The model under review builds one solid part; all positions refer to its coordinate system, in mm. A direction names the side the tool comes from. Give positions to 0.01 mm unless a question says otherwise; leave off trailing zeros. Order: outer loops, then holes, each group sorted by start corner. A loop starts at its lowest first (then second) coordinate and runs counter-clockwise, first axis right, second up. Notation, with made-up numbers: (-10.75, 48) - (6.25, 48) arc R18 cw to (6.25, 80) - close; hole circle Ø11 at (55, 84.5). An arc over 180 degrees is marked (long way). Put each result on its own line as item: value.
```python
from build123d import *

# Parameters (mm, degrees)
F0_R     = 3.175
F0_R_2   = 9.525
F1_DEPTH = 25.4
F2_R     = 5.08
F3_SIZE  = 1.5875
F4_R     = 1.5875
F5_SIZE  = 1.5875


with BuildPart() as f1:
    # F0 (on Top) → F1 (new body)
    with BuildSketch(Plane.XY):
        Polygon((0, 0), (-25.4, 0), (-25.4, -25.4), (50.8, -25.4), (50.8, 38.1), (25.4, 38.1), (25.4, 12.7), (0, 12.7), align=None)
        with Locations((-12.7, -12.7)):
            Circle(F0_R, mode=Mode.SUBTRACT)
        with Locations((25.4, 0)):
            Circle(F0_R_2, mode=Mode.SUBTRACT)
    extrude(amount=F1_DEPTH)

    # F2
    f2_edges = [f1.edges().sort_by_distance(p)[0] for p in [
        (50.8, 38.1, 12.7),
        (25.4, 38.1, 12.7),
        (25.4, 12.7, 12.7),
        (0, 12.7, 12.7),
        (0, 0, 12.7),
        (-25.4, 0, 12.7),
        (-25.4, -25.4, 12.7),
        (50.8, -25.4, 12.7),
    ]]
    fillet(f2_edges, radius=F2_R)

    # F3
    f3_edges = [f1.edges().sort_by_distance(p)[0] for p in [
        (15.875, 0, 25.4),
    ]]
    chamfer(f3_edges, length=F3_SIZE)

    # F4
    f4_edges = [f1.edges().sort_by_distance(p)[0] for p in [
        (-25.4, -12.7, 25.4),
        (12.7, -25.4, 0),
    ]]
    fillet(f4_edges, radius=F4_R)

    # F5
    f5_edges = [f1.edges().sort_by_distance(p)[0] for p in [
        (15.875, 0, 0),
    ]]
    chamfer(f5_edges, length=F5_SIZE)


solid = f1.part
```
(1) Take a section at D-D, the plane y = 20.5. Write out the cut boundary in (x, z) (1 decimal), then the cut area to 3 significant figures.
The answers:
outline: (25.4, 1.6) arc R1.6 ccw to (27, 0) - (49.2, 0) arc R1.6 ccw to (50.8, 1.6) - (50.8, 23.8) arc R1.6 ccw to (49.2, 25.4) - (27, 25.4) arc R1.6 ccw to (25.4, 23.8) - close
area: 643 mm^2
(2) Take a section at B-B, the plane y = -12.7. Write out the cut boundary in (x, z) (1 decimal).
The answers:
outline: (-25.4, 1.6) arc R1.6 ccw to (-23.8, 0) - (-15.9, 0) - (-15.9, 25.4) - (-23.8, 25.4) arc R1.6 ccw to (-25.4, 23.8) - close; (-9.5, 0) - (49.2, 0) arc R1.6 ccw to (50.8, 1.6) - (50.8, 23.8) arc R1.6 ccw to (49.2, 25.4) - (-9.5, 25.4) - close
(3) The part is to be moulded in two halves that separate along X. For faces 5 (the cylindrical face through (-23.872, -1.449, 12.856)), 6 (the cylindrical face through (15.884, 0.419, 12.544)), 7 (the cylindrical face through (50.35, 6.72, 0.48)), say which applies: pulls with the +X half, pulls with the -X half, needs draft (parallel to the pull), parting line crosses it, or undercut.
The answers:
face 5: pulls with the -X half
face 6: undercut
face 7: pulls with the +X half
(4) For faces 1 (the cylindrical face through (-12.81, -0.48, 24.95)), 2 (the flat face through (13, 12.7, 13)), 3 (the cylindrical face through (-12.81, -0.45, 0.48)), 4 (the cylindrical face through (13.16, -24.95, 0.48)), list the 3-axis set-ups (+Z, -Z, +X, -X, +Y, -Y) from which the entire face can be reached by the end or side of a thin tool; tool diameter is ignored.
The answers:
face 1: +Z, -X, +Y
face 2: +Z, -Z, -X, +Y
face 3: -Z, -X, +Y
face 4: -Z, +X, -X, -Y
(5) Take a section at C-C, the plane x = -12.7. Write out the cut boundary in (y, z) (1 decimal).
The answers:
outline: (-25.4, 1.6) arc R1.6 ccw to (-23.8, 0) - (-15.9, 0) - (-15.9, 25.4) - (-23.8, 25.4) arc R1.6 ccw to (-25.4, 23.8) - close; (-9.5, 0) - (-1.6, 0) arc R1.6 ccw to (0, 1.6) - (0, 23.8) arc R1.6 ccw to (-1.6, 25.4) - (-9.5, 25.4) - close
(6) Clearance check with flat-ended pins moving along their axes: pin 1 Ø12 at (x, z) = (-14.5, 12.5) entering from +Y; pin 2 Ø3 at (y, z) = (6.5, 8.5) entering from -X; pin 3 Ø4.5 at (y, z) = (22.5, 7.5) entering from -X; pin 4 Ø15 at (x, y) = (25.4, 0) entering from -Z. State where each tip first meets the part, or that it passes through.
The answers:
pin 1: y = 0
pin 2: x = 0
pin 3: x = 25.4
pin 4: through
(7) Wall thickness on L1, parallel to Y at x = -12.7, z = 8.25 (3 decimals); L2, parallel to Y at x = 10, z = 19.5; L3, parallel to X at y = 4.5, z = 19.5: over which ranges is each line inside the solid? List them lowest first.
The answers:
L1: -25.4 to -15.875, -9.525 to 0
L2: -25.4 to 12.7
L3: -0.03 to 17.01, 33.79 to 50.8
(8) Take a section at A-A, the plane z = 6.75. Write out the cut boundary in (x, y) (3 decimals), then the cut area to 3 significant figures.
The answers:
outline: (-25.4, -20.32) arc R5.08 ccw to (-20.32, -25.4) - (45.72, -25.4) arc R5.08 ccw to (50.8, -20.32) - (50.8, 33.02) arc R5.08 ccw to (45.72, 38.1) - (30.48, 38.1) arc R5.08 ccw to (25.4, 33.02) - (25.4, 17.78) arc R5.08 cw to (20.32, 12.7) - (5.08, 12.7) arc R5.08 ccw to (0, 7.62) - (0, 5.08) arc R5.08 cw to (-5.08, 0) - (-20.32, 0) arc R5.08 ccw to (-25.4, -5.08) - close; hole circle Ø6.35 at (-12.7, -12.7); hole circle Ø19.05 at (25.4, 0)
area: 2,890 mm^2
